from build123d import *

# Parameters (mm, degrees)
F1_DEPTH = 8
F2_R     = 1.55
F3_DEPTH = 12.5
F4_DEPTH = 1
F6_DEPTH = 25
F8_DEPTH = 25
F9_R     = 3
F10_R    = 3
F11_R    = 0.5


with BuildPart() as f1:
    # F0 (on Top) → F1 (new body)
    with BuildSketch(Plane.XY):
        with BuildLine():
            ThreePointArc((1.5, 3.7619808612), (0, -4.05), (-1.5, 3.7619808612))
            Line((-1.5, 3.7619808612), (-1.5, 7.909013845))
            Line((-1.5, 7.909013845), (-1.5, 9.7619808612))
            Line((-1.5, 9.7619808612), (-3.4838211723, 9.7619808612))
            Line((-3.4838211723, 9.7619808612), (-3.4838211723, 7.2570992855))
            ThreePointArc((-3.4838211723, 7.2570992855), (0, -8.05), (3.4838211723, 7.2570992855))
            Line((3.4838211723, 7.2570992855), (3.4838211723, 9.7619808612))
            Line((3.4838211723, 9.7619808612), (1.5, 9.7619808612))
            Line((1.5, 9.7619808612), (1.5, 7.909013845))
            Line((1.5, 7.909013845), (1.5, 3.7619808612))
        make_face()
    extrude(amount=F1_DEPTH)

    # F2 (on Right) → F3 (cut, symmetric)
    with BuildSketch(Plane.YZ):
        with Locations((7.2570992855, 4)):
            Circle(F2_R)
    extrude(amount=F3_DEPTH, both=True, mode=Mode.SUBTRACT)

    # F4 (add): faces of the model
    f4_faces = [f1.faces().sort_by_distance(p)[0] for p in [
        (2.4919105861, 9.7619808612, 4),
        (-2.4919105861, 9.7619808612, 4),
    ]]
    extrude(f4_faces, amount=F4_DEPTH)

    # F5 (on face) → F6 (cut)
    with BuildSketch(Plane.YZ.offset(3.4838211723)):
        with BuildLine():
            Line((7.2570992855, 5.55), (7.2570992855, 7))
            ThreePointArc((7.2570992855, 7), (4.2570992855, 4), (7.2570992855, 1))
            Line((7.2570992855, 1), (7.2570992855, 2.45))
            ThreePointArc((7.2570992855, 2.45), (8.3531147963, 2.9039844892), (8.8070992855, 4))
            ThreePointArc((8.8070992855, 4), (8.3531147963, 5.0960155108), (7.2570992855, 5.55))
        make_face()
    extrude(amount=F6_DEPTH, mode=Mode.SUBTRACT)

    # F7 (on face) → F8 (cut)
    with BuildSketch(Plane(origin=(-3.4838211723, 0, 0), x_dir=(0, -1, 0), z_dir=(-1, 0, 0))):
        with BuildLine():
            ThreePointArc((-7.2570992855, 1), (-5.1357789419, 1.8786796564), (-4.2570992855, 4))
            ThreePointArc((-4.2570992855, 4), (-5.1357789419, 6.1213203436), (-7.2570992855, 7))
            Line((-7.2570992855, 7), (-7.2570992855, 5.55))
            ThreePointArc((-7.2570992855, 5.55), (-8.3531147963, 5.0960155108), (-8.8070992855, 4))
            ThreePointArc((-8.8070992855, 4), (-8.3531147963, 2.9039844892), (-7.2570992855, 2.45))
            Line((-7.2570992855, 2.45), (-7.2570992855, 1))
        make_face()
    extrude(amount=F8_DEPTH, mode=Mode.SUBTRACT)

    # F9
    f9_edges = [f1.edges().sort_by_distance(p)[0] for p in [
        (2.491911, 10.761981, 8),
        (2.491911, 10.761981, 0),
    ]]
    fillet(f9_edges, radius=F9_R)

    # F10
    f10_edges = [f1.edges().sort_by_distance(p)[0] for p in [
        (-2.491911, 10.761981, 8),
        (-2.491911, 10.761981, 0),
    ]]
    fillet(f10_edges, radius=F10_R)

    # F11
    f11_edges = [f1.edges().sort_by_distance(p)[0] for p in [
        (-3.483821, 9.883301, 7.12132),
        (-3.483821, 7.50954, 8),
        (0, -8.05, 8),
        (3.483821, 7.50954, 8),
        (3.483821, 9.883301, 7.12132),
        (3.483821, 10.761981, 4),
        (-3.483821, 10.761981, 4),
        (-3.483821, 9.883301, 0.87868),
        (-3.483821, 7.50954, 0),
        (0, -8.05, 0),
        (3.483821, 7.50954, 0),
        (3.483821, 9.883301, 0.87868),
    ]]
    fillet(f11_edges, radius=F11_R)


solid = f1.part
Build history of the part. All positions in model axes, mm. A direction names the side the tool comes from. Round coordinates to 2 decimals unless told otherwise and drop trailing zeros. Write each loop counter-clockwise with the first axis right and the second up, starting at its lowest first coordinate (ties: lowest second). Pieces come first, ordered by that corner, then holes. Notation, with made-up numbers: M 14,-18 L 58,-18 A21 cw 58,-2 Z; hole C 75.5,25.5 d7. An arc over 180 degrees is marked long. Answer as a JSON object with one key per item and string values. Group by question number.
(1) Cut at B-B (x = 0). Give the cut face in (y, z).
(2) Which spindle directions (+Z, -Z, +X, -X, +Y, -Y) get a long thin tool onto all of the face, cutting with end or side? Do faces 1 (the flat face through (-3.484, 9, 3)), 2 (the flat face through (3.484, 8, 6)), 3 (the flat face through (-1.5, 5.7, 4.8)), 4 (the cylindrical face through (2, 10, 7)). Say none if no direction does.
(3) Cut at C-C (x = 2). Give the number of separate pieces and of enclosed holes in the cut face, and give its area (3 significant figures).
(4) Flat gauge pins, fed straight in: pin 1 (3.5 mm diameter, centred on y = 5.5, z = 5.5, fed in from -X); pin 2 (5 mm diameter, centred on x = 0, y = 0, fed in from +Z); pin 3 (3 mm diameter, centred on y = 7, z = 5, fed in from +X); pin 4 (1.8 mm diameter, centred on y = 6, z = 3.5, fed in from -X). Where does each tip first touch, or does it go through?
(5) Drill centre lines: L1, parallel to X at y = 9.75, z = 5.75; L2, parallel to Y at x = 2.4, z = 4; L3, parallel to Y at x = 2.1, z = 4. Where is each one in solid material? Low to high.
(6) Mould opens along Y. For faces 5 (the cylindrical face through (-0.304, -8.044, 3.951)), 6 (the flat face through (-3, -3, 0)), 7 (the cylindrical face through (0.157, -4.047, 3.944)), 8 (the cylindrical face through (-2, 10, 7)) say: pulls with the +Y half, pulls with the -Y half, needs draft (parallel to the pull), parting line crosses it, or undercut.
(7) Cut at A-A (z = 4.5). Give the cut face in (x, y).
Responses:
{
 "1": {"outline": "M -8.05,0.5 A0.5 ccw -7.55,0 L -4.05,0 L -4.05,8 L -7.55,8 A0.5 ccw -8.05,7.5 Z"},
 "2": {"face 1": "-X, +Y", "face 2": "+X, +Y", "face 3": "+Z, -Z, +Y", "face 4": "+Z, +X, -X, +Y"},
 "3": {"separate pieces": "2", "enclosed holes": "1", "area": "80.6 mm2"},
 "4": {"pin 1": "stops at x = -7.12", "pin 2": "passes through", "pin 3": "stops at x = 3.48", "pin 4": "stops at x = -3.48"},
 "5": {"L1": "x = -3.48 to -1.5, 1.5 to 3.48", "L2": "y = -7.68 to -3.26, 3.26 to 5.71, 8.81 to 10.76", "L3": "y = -7.77 to -3.46, 3.46 to 5.71, 8.81 to 10.76"},
 "6": {"face 5": "parting line crosses it", "face 6": "needs draft", "face 7": "undercut", "face 8": "pulls with the +Y half"},
 "7": {"outline": "M -6.81,4.3 A8.05 ccw long 6.81,4.3 L 3.48,4.3 L 3.48,5.79 L 1.5,5.79 L 1.5,3.76 A4.05 cw long -1.5,3.76 L -1.5,5.79 L -3.48,5.79 L -3.48,4.3 Z; M -3.48,8.72 L -1.5,8.72 L -1.5,10.76 L -2.98,10.76 A0.5 ccw -3.48,10.26 Z; M 1.5,8.72 L 3.48,8.72 L 3.48,10.26 A0.5 ccw 2.98,10.76 L 1.5,10.76 Z"}
}
